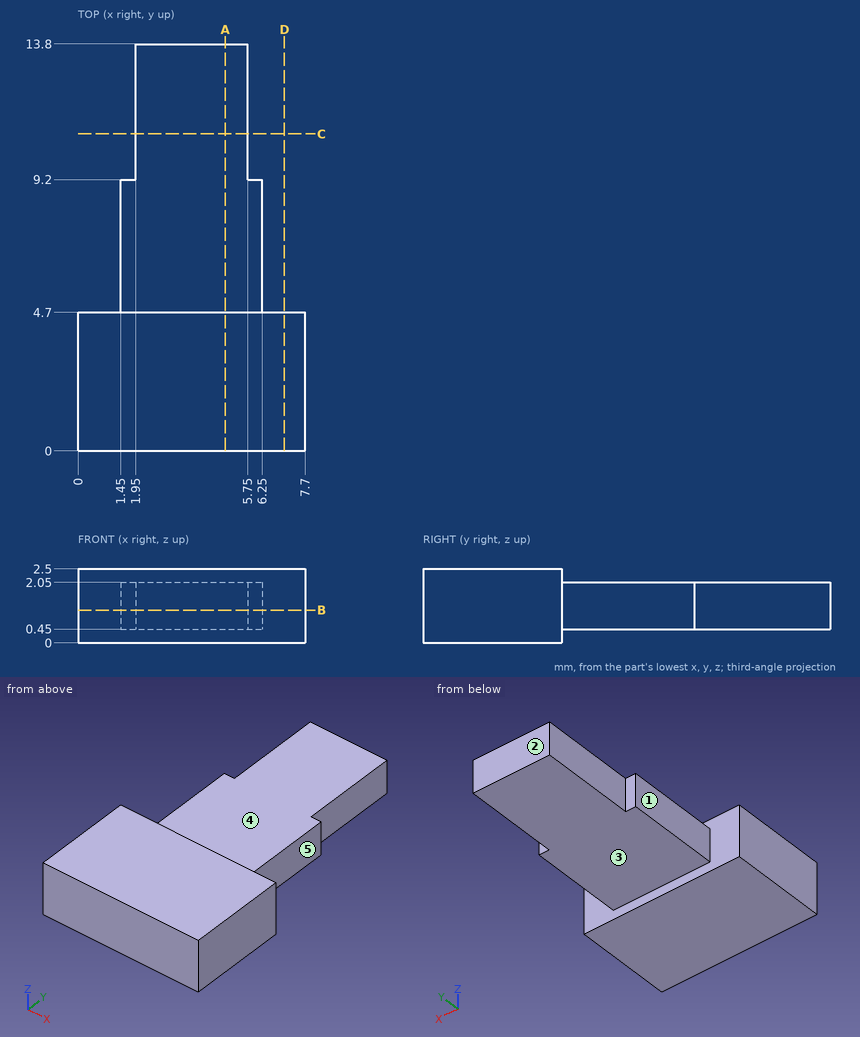
Here's the drawing with two shaded views (mm, measured from the low corner). I have some questions. A direction names the side the tool comes from. Give positions to 0.01 mm unless a question says otherwise; leave off trailing zeros. Write each loop counter-clockwise with the first axis right and the second up, starting at its lowest first coordinate (ties: lowest second). Pieces come first, ordered by that corner, then holes. Notation, with made-up numbers: (-37.5, 23.5) -> (-3.5, 23.5) arc R26 ccw to (-3.5, 49.5) -> close; hole circle Ø3 at (42, 88). An arc over 180 degrees is marked (long way). Use one line per item in the form item = value.
1) On a 3-axis mill with a long thin cutter (end or side, diameter ignored), from which of +Z, -Z, +X, -X, +Y, -Y can I reach the whole of each face in a straight line? I mean the marked faces 1, 2, 3, 4 and 5. Say none if no direction works.
Verdict:
face_1 = +Z, -Z, -X, +Y
face_2 = +Z, -Z, +X, -X, +Y
face_3 = -Z, +X, -X, +Y
face_4 = +Z, +X, -X, +Y
face_5 = +Z, -Z, +X, +Y
2) Suppose I cut it at B-B (z = 1.1). Please give me the cut outline in (x, y).
Verdict:
outline = (0, 0) -> (7.7, 0) -> (7.7, 4.7) -> (6.25, 4.7) -> (6.25, 9.2) -> (5.75, 9.2) -> (5.75, 13.8) -> (1.95, 13.8) -> (1.95, 9.2) -> (1.45, 9.2) -> (1.45, 4.7) -> (0, 4.7) -> close
3) Suppose I cut it at D-D (x = 7). Please give me the cut outline in (y, z), and give its area (4 significant figures).
Verdict:
outline = (0, 0) -> (4.7, 0) -> (4.7, 2.5) -> (0, 2.5) -> close
area = 11.75 mm2
4) If I drill on L1, parallel to Y at x = 7, z = 2.2; L2, parallel to Z at x = 3.75, y = 7.25; L3, parallel to Y at x = 6, z = 1.9, over which ranges is the centre line in solid material (lowest first)? Write a range as [from, to].
Verdict:
L1 = [0, 4.7]
L2 = [0.45, 2.05]
L3 = [0, 9.2]
5) Suppose I cut it at A-A (x = 5). Please give me the cut outline in (y, z).
Verdict:
outline = (0, 0) -> (4.7, 0) -> (4.7, 0.45) -> (13.8, 0.45) -> (13.8, 2.05) -> (4.7, 2.05) -> (4.7, 2.5) -> (0, 2.5) -> close
6) Suppose I cut it at C-C (y = 10.75). Please give me the cut outline in (x, z), and give its area (3 significant figures).
Verdict:
outline = (1.95, 0.45) -> (5.75, 0.45) -> (5.75, 2.05) -> (1.95, 2.05) -> close
area = 6.08 mm2
7) I'm going to push flat-ended pins straight in: pin 1 (0.5 mm diameter, centred on y = 11.5, z = 1.5, fed in from +X); pin 2 (1.3 mm diameter, centred on y = 7.5, z = 1, fed in from +X); pin 3 (0.8 mm diameter, centred on y = 10.5, z = 1.5, fed in from -X); pin 4 (3 mm diameter, centred on x = 2, y = 5.5, fed in from +Z). Where does each tip first touch, or does it pass through?
Verdict:
pin_1 = 5.75
pin_2 = 6.25
pin_3 = 1.95
pin_4 = 2.5
